Build history of the part. All positions in model axes, mm. Round coordinates to 2 decimals unless told otherwise and drop trailing zeros. Order: outer loops, then holes, each group sorted by start corner. A loop starts at its lowest first (then second) coordinate and runs counter-clockwise, first axis right, second up. Notation, with made-up numbers: (61, 64.5) -> (97, 64.5) arc R14 cw to (97, 89.5) -> close; hole circle Ø10 at (27, -29.75). An arc over 180 degrees is marked (long way). Write item = value, one per line.
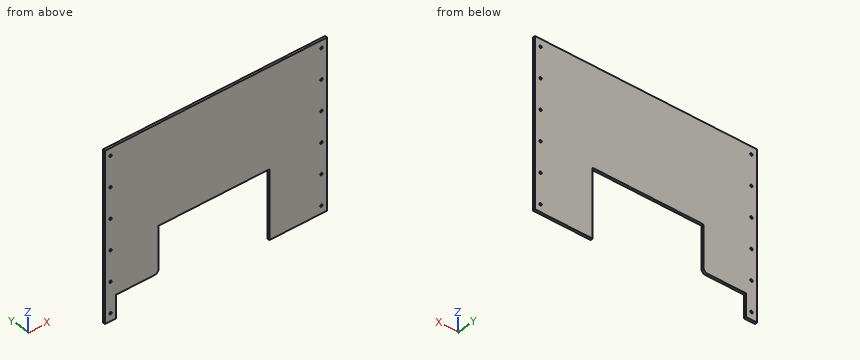
from build123d import *

# Parameters (mm, degrees)
BOSS_EXTRUDE1_DEPTH = 3.18
SKETCH2_R           = 1.65
CUT_EXTRUDE1_DEPTH  = 10
FILLET1_R           = 5


with BuildPart() as part:
    # Sketch1 → Boss-Extrude1 (new body)
    with BuildSketch(Plane(origin=(0, 0, 0), x_dir=(1, 0, 0), z_dir=(0, 1, 0))):
        Polygon((72.127496387, 91.855323554), (72.127496387, 1.855323554), (-77.872503613, 1.855323554), (-77.872503613, 61.855323554), (-134.872503613, 61.855323554), (-134.872503613, 91.855323554), (-150, 91.855323554), (-150, -128.144676446), (150, -128.144676446), (150, 91.855323554), align=None)
    extrude(amount=BOSS_EXTRUDE1_DEPTH)

    # Sketch2 → Cut-Extrude1 (cut)
    with BuildSketch(Plane(origin=(0, 3.18, 0), x_dir=(1, 0, 0), z_dir=(0, 1, 0))):
        with Locations(Location((-142.5, 81.855323554, 0), (0, 0, 270))):
            Circle(SKETCH2_R)
        with Locations(Location((-142.5, 41.855323554, 0), (0, 0, 270))):
            Circle(SKETCH2_R)
        with Locations(Location((-142.5, 1.855323554, 0), (0, 0, 270))):
            Circle(SKETCH2_R)
        with Locations(Location((-142.5, -38.144676446, 0), (0, 0, 270))):
            Circle(SKETCH2_R)
        with Locations(Location((-142.5, -78.144676446, 0), (0, 0, 270))):
            Circle(SKETCH2_R)
        with Locations(Location((-142.5, -118.144676446, 0), (0, 0, 270))):
            Circle(SKETCH2_R)
        with Locations(Location((142.5, 81.855323554, 0), (0, 0, 270))):
            Circle(SKETCH2_R)
        with Locations(Location((142.5, 41.855323554, 0), (0, 0, 270))):
            Circle(SKETCH2_R)
        with Locations(Location((142.5, 1.855323554, 0), (0, 0, 270))):
            Circle(SKETCH2_R)
        with Locations(Location((142.5, -38.144676446, 0), (0, 0, 270))):
            Circle(SKETCH2_R)
        with Locations(Location((142.5, -78.144676446, 0), (0, 0, 270))):
            Circle(SKETCH2_R)
        with Locations(Location((142.5, -118.144676446, 0), (0, 0, 270))):
            Circle(SKETCH2_R)
    extrude(amount=-CUT_EXTRUDE1_DEPTH, mode=Mode.SUBTRACT)

    # Fillet1
    fillet1_edges = [part.edges().sort_by_distance(p)[0] for p in [
        (-77.872503613, 1.59, -61.855323554),
    ]]
    fillet(fillet1_edges, radius=FILLET1_R)


solid = part.part
Q1. Cut at B-B, the plane y = 2.5. Give the number of separate pieces and of enclosed holes in the cut face, and give its area (3 significant figures).
Check values:
separate_pieces = 1
enclosed_holes = 12
area = 50,700 mm²
Q2. Flat gauge pin, fed straight in: pin 1 (3 mm diameter, centred on x = -142.5, z = 78.14, fed in from -Y) (3 decimals). Where does the tip first touch, or does it go through?
Check values:
pin_1 = through
Q3. Cut at C-C, the plane z = -71.5. List the corners of the cut face in (x, y).
Check values:
outline = (-150, 0) -> (-134.87, 0) -> (-134.87, 3.18) -> (-150, 3.18) -> close; (72.13, 0) -> (150, 0) -> (150, 3.18) -> (72.13, 3.18) -> close
Q4. Cut at D-D, the plane x = 29. List the corners of the cut face in (y, z).
Check values:
outline = (0, -1.86) -> (3.18, -1.86) -> (3.18, 128.14) -> (0, 128.14) -> close
Q5. Probe probe 1 along X at (y, z) = (2.35, -7); probe 2 along Z at (x, y) = (-120, 1.55); probe 3 along X at (y, z) = (1.8, -76.5). List the from-to ranges inside material, lowest first.
Check values:
probe_1 = -150 to -77.87, 72.13 to 150
probe_2 = -61.86 to 128.14
probe_3 = -150 to -134.87, 72.13 to 150
Q6. Cut at A-A, the plane z = -13.5. List the corners of the cut face in (x, y), and give its area (3 significant figures).
Check values:
outline = (-150, 0) -> (-77.87, 0) -> (-77.87, 3.18) -> (-150, 3.18) -> close; (72.13, 0) -> (150, 0) -> (150, 3.18) -> (72.13, 3.18) -> close
area = 477 mm²
